Verification items for the finished model (mm, model axes). Face numbers are marked on the shaded views. Round coordinates to 2 decimals unless told otherwise and drop trailing zeros. Loops run counter-clockwise (first coordinate to the right, second up) from the corner with the lowest first, then second, coordinate; pieces in that order, holes last. Notation, with made-up numbers: M 73,-9 L 103,-9 A19 ccw 103,-4 Z; hole C 20,58.5 d9. An arc over 180 degrees is marked long. Answer as CSV lines item,"result".
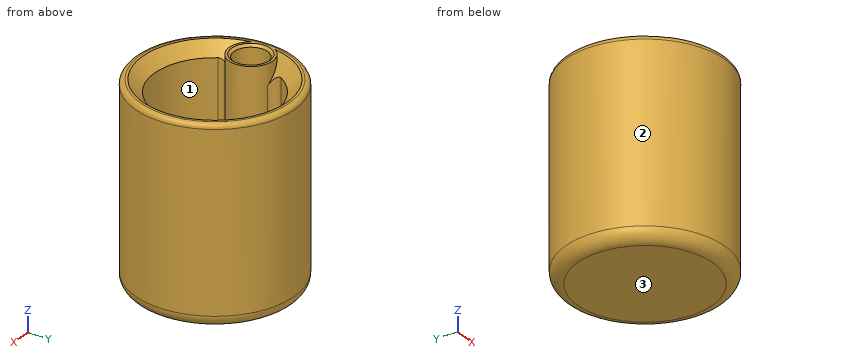
```python
from build123d import *

# Parameters (mm, degrees)
SKETCH_R            = 33
PAD_DEPTH           = 80
HOLE_D              = 50
HOLE_DEPTH          = 70
HOLE_CSINK_D        = 60
HOLE_CSINK_ANGLE    = 90
SKETCH002_R         = 9
PAD001_DEPTH        = 80
HOLE001_D           = 14
HOLE001_DEPTH       = 65.875644
HOLE001_CSINK_D     = 16
HOLE001_CSINK_ANGLE = 90
HOLE001_TIPS_R      = 7
FILLET_R            = 3
FILLET001_R         = 2
FILLET002_R         = 5


with BuildPart() as part:
    # Sketch → Pad (new body)
    with BuildSketch(Plane.XY):
        Circle(SKETCH_R)
    extrude(amount=PAD_DEPTH)

    # Hole
    with Locations(Plane.XY.offset(80)):
        with Locations((0, 0)):
            CounterSinkHole(HOLE_D / 2, HOLE_CSINK_D / 2, depth=HOLE_DEPTH, counter_sink_angle=HOLE_CSINK_ANGLE)

    # Sketch002 (on Face3 of Hole) → Pad001 (join)
    with BuildSketch(Plane.XY.offset(80)):
        with Locations((-22, 0)):
            Circle(SKETCH002_R)
    extrude(amount=-PAD001_DEPTH)

    # Hole001
    with Locations(Plane.XY.offset(80)):
        with Locations((-22, 0)):
            CounterSinkHole(HOLE001_D / 2, HOLE001_CSINK_D / 2, depth=HOLE001_DEPTH, counter_sink_angle=HOLE001_CSINK_ANGLE)

    # Hole001 tips → Hole001 tip 1 section 0
    with BuildSketch(Plane.XY.offset(14.124356), mode=Mode.PRIVATE) as hole001_tip_1_s0:
        with Locations((-22, 0)):
            Circle(HOLE001_TIPS_R)
    loft([hole001_tip_1_s0.sketch, Vertex(-22, 0, 2)], mode=Mode.SUBTRACT)

    # Fillet
    fillet_edges = [part.edges().sort_by_distance(p)[0] for p in [
        (-23.363636, -8.896094, 42.5),
        (-23.363636, 8.896094, 42.5),
    ]]
    fillet(fillet_edges, radius=FILLET_R)

    # Fillet001
    fillet001_edges = [part.edges().sort_by_distance(p)[0] for p in [
        (-33, 0, 80),
    ]]
    fillet(fillet001_edges, radius=FILLET001_R)

    # Fillet002
    fillet002_edges = [part.edges().sort_by_distance(p)[0] for p in [
        (-33, 0, 0),
    ]]
    fillet(fillet002_edges, radius=FILLET002_R)


solid = part.part
```
1) Material ranges on probe 1 along X at (y, z) = (2.5, 56); probe 2 along X at (y, z) = (-3, 44); probe 3 along Z at (x, y) = (-18.5, -9.5), recorded low to high.
Here are the results:
probe 1,"x = -32.91 to -28.54, -15.46 to -13.35, 24.87 to 32.91"
probe 2,"x = -32.86 to -28.32, -15.68 to -13.51, 24.82 to 32.86"
probe 3,"z = 0 to 10"
2) Go/stop test with flat-tipped pins: pin 1 (1.5 mm diameter, centred on x = -25.5, z = 28, fed in from -Y); pin 2 (3 mm diameter, centred on x = 16, z = 67, fed in from +Y); pin 3 (5 mm diameter, centred on x = -12.5, z = 41, fed in from +Y). Record where each tip stops, or that it passes through.
Here are the results:
pin 1,"stops at y = -21.83"
pin 2,"stops at y = 29.64"
pin 3,"stops at y = 31.45"
3) Draft check along X on the marked faces 1, 2 and 3. Enter one of: +X half, -X half, draft (parallel to the pull), parting line (faces both ways), or undercut.
Here are the results:
face 1,"undercut"
face 2,"parting line"
face 3,"draft"
4) Section check A-A (x = 0). Record the cut outline in (y, z).
Here are the results:
outline,"M -33,5 A5 ccw -28,0 L 28,0 A5 ccw 33,5 L 33,78 A2 ccw 31,80 L 30,80 L 25,75 L 25,10 L -25,10 L -25,75 L -30,80 L -31,80 A2 ccw -33,78 Z"
5) Section check B-B (z = 55). State how many separate pieces and enclosed holes the cut face has, plus the area to 3 significant figures.
Here are the results:
separate pieces,"1"
enclosed holes,"2"
area,"1,480 mm^2"
